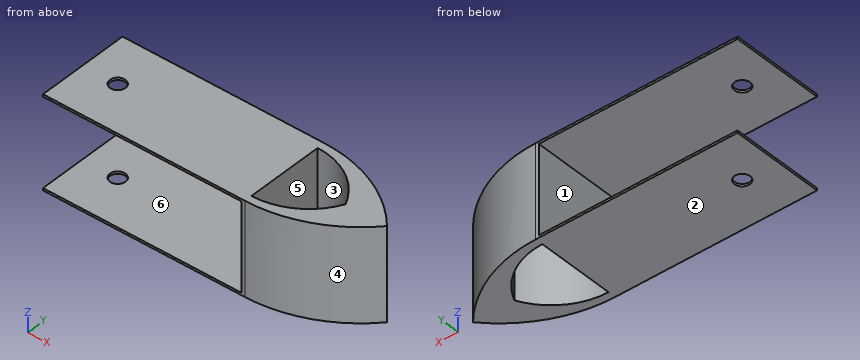
```python
from build123d import *

# Parameters (mm, degrees)
RESSALTO_EXTRUS_O1_DEPTH   = 60
CORTE_EXTRUS_O1_DEPTH      = 148.170653102
CORTE_EXTRUS_O1_DEPTH_BACK = 148.170653102
CORTE_EXTRUS_O2_DEPTH      = 148.170653102
CORTE_EXTRUS_O2_DEPTH_BACK = 148.170653102
ESBO_O5_W                  = 126
ESBO_O5_H                  = 57
ESBO_O6_W                  = 57
ESBO_O6_H                  = 60
CORTE_EXTRUS_O3_DEPTH      = 57
CORTE_EXTRUS_O4_DEPTH      = 148.170653102
CORTE_EXTRUS_O4_DEPTH_BACK = 57
ESBO_O7_R                  = 5


with BuildPart() as part:
    # Esboço1 → Ressalto-extrusão1 (new body)
    with BuildSketch(Plane.XY):
        with BuildLine():
            Line((65, 30), (-65, 30))
            Line((-65, 30), (-65, -30))
            Line((-65, -30), (65, -30))
            ThreePointArc((65, -30), (101.246012625, -22.148036763), (130.993133921, 0))
            ThreePointArc((130.993133921, 0), (101.246012625, 22.148036763), (65, 30))
        make_face()
    extrude(amount=RESSALTO_EXTRUS_O1_DEPTH)

    # Esboço3 → Corte-extrusão1 (cut, two sides: drawn at the far end of the back side and taken through both)
    with BuildSketch(Plane.XY.offset(-CORTE_EXTRUS_O1_DEPTH_BACK)):
        with BuildLine():
            Line((65, 25), (65, -25))
            ThreePointArc((65, -25), (88.305470739, -18.221231084), (104.339291624, 0))
            ThreePointArc((104.339291624, 0), (88.305470739, 18.221231084), (65, 25))
        make_face()
    extrude(amount=CORTE_EXTRUS_O1_DEPTH + CORTE_EXTRUS_O1_DEPTH_BACK, mode=Mode.SUBTRACT)

    # Esboço5 → Corte-extrusão2 (cut, two sides: drawn at the far end of the back side and taken through both)
    with BuildSketch(Plane(origin=(0, 0, 0), x_dir=(1, 0, 0), z_dir=(0, 1, 0)).offset(-CORTE_EXTRUS_O2_DEPTH_BACK)):
        with Locations((0, -30)):
            Rectangle(ESBO_O5_W, ESBO_O5_H)
    extrude(amount=CORTE_EXTRUS_O2_DEPTH + CORTE_EXTRUS_O2_DEPTH_BACK, mode=Mode.SUBTRACT)

    # Esboço6 → Corte-extrusão3 (cut)
    with BuildSketch(Plane(origin=(-63, 0, 0), x_dir=(0, 0, -1), z_dir=(1, 0, 0))):
        with Locations((-30, 0)):
            Rectangle(ESBO_O6_W, ESBO_O6_H)
    extrude(amount=-CORTE_EXTRUS_O3_DEPTH, mode=Mode.SUBTRACT)

    # Esboço7 → Corte-extrusão4 (cut, two sides: drawn at the far end of the back side and taken through both)
    with BuildSketch(Plane.XY.offset(-CORTE_EXTRUS_O4_DEPTH_BACK)):
        with Locations((-42.467037106, 0)):
            Circle(ESBO_O7_R)
    extrude(amount=CORTE_EXTRUS_O4_DEPTH + CORTE_EXTRUS_O4_DEPTH_BACK, mode=Mode.SUBTRACT)


solid = part.part
```
The model under review builds one solid part; all positions refer to its coordinate system, in mm. Face numbers are marked on the shaded views. A direction names the side the tool comes from. Round coordinates to 2 decimals unless told otherwise and drop trailing zeros. Write each loop counter-clockwise with the first axis right and the second up, starting at its lowest first coordinate (ties: lowest second). Pieces come first, ordered by that corner, then holes. Notation, with made-up numbers: (70, 60) - (97, 60) arc R24 ccw to (97, 71) - close; hole circle Ø4 at (40.5, 67). An arc over 180 degrees is marked (long way). Answer as CSV lines item,"result". Start each with the question number.
(1) We need section D-D on x = 93.5. State the section outline as (y, z) points, plus the area to 3 significant figures.
(2) To check wall thickness, follow line 1 (X direction, y = 0, z = 59.1); line 2 (Z direction, x = 42, y = 6); line 3 (X direction, y = 11.5, z = 18). State the ranges of each line that lie inside material, in increasing order.
(3) For pin 1 Ø4 at (x, z) = (95.5, 47.5) entering from +Y; pin 2 Ø1.5 at (x, z) = (100.5, 20) entering from -Y; pin 3 Ø2 at (y, z) = (19.5, 27) entering from +X, all flat-tipped, find the tip position at first contact; note any pin that passes through.
(4) We need section C-C on y = 18.5. State the section outline as (x, z) points, plus the area to 3 significant figures.
(5) We need section A-A on z = 42. State the section outline as (x, y) points.
(6) For the marked faces 1, 2 and 3, list the 3-axis set-ups (+Z, -Z, +X, -X, +Y, -Y) from which the entire face can be reached by the end or side of a thin tool; tool diameter is ignored.
(7) Draft analysis for pull direction Y (two halves, no side actions). For the marked faces 4, 5 and 6, state which applies: pulls with the +Y half, pulls with the -Y half, needs draft (parallel to the pull), parting line crosses it, or undercut.
(8) We need section B-B on y = -3. State the section outline as (x, z) points.
Worked answers:
1,outline,"(-25.23, 0) - (-14.35, 0) - (-14.35, 60) - (-25.23, 60) - close; (14.35, 0) - (25.23, 0) - (25.23, 60) - (14.35, 60) - close"
1,area,"1,310 mm²"
2,line 1,"-65 to -47.47, -37.47 to 65, 104.34 to 130.99"
2,line 2,"0 to 1.5, 58.5 to 60"
2,line 3,"63 to 65, 96.48 to 118.84"
3,pin 1,"y = 25.23"
3,pin 2,"y = -22.81"
3,pin 3,"x = 108.38"
4,outline,"(-65, 0) - (65, 0) - (65, 60) - (-65, 60) - (-65, 58.5) - (63, 58.5) - (63, 1.5) - (-65, 1.5) - close; (87.86, 0) - (108.38, 0) - (108.38, 60) - (87.86, 60) - close"
4,area,"1,740 mm²"
5,outline,"(63, -30) - (65, -30) arc R87.58 ccw to (130.99, 0) arc R87.58 ccw to (65, 30) - (63, 30) - close; hole (65, -25) arc R43.45 ccw to (104.34, 0) arc R43.45 ccw to (65, 25) - close"
6,face 1,"-X, +Y, -Y"
6,face 2,"-Z, +X, -X, +Y, -Y"
6,face 3,"+Z, -Z"
7,face 4,"pulls with the -Y half"
7,face 5,"undercut"
7,face 6,"needs draft"
8,outline,"(-65, 0) - (-46.47, 0) - (-46.47, 1.5) - (-65, 1.5) - close; (-65, 58.5) - (-46.47, 58.5) - (-46.47, 60) - (-65, 60) - close; (-38.47, 0) - (65, 0) - (65, 60) - (-38.47, 60) - (-38.47, 58.5) - (63, 58.5) - (63, 1.5) - (-38.47, 1.5) - close; (102.79, 0) - (128.25, 0) - (128.25, 60) - (102.79, 60) - close"
